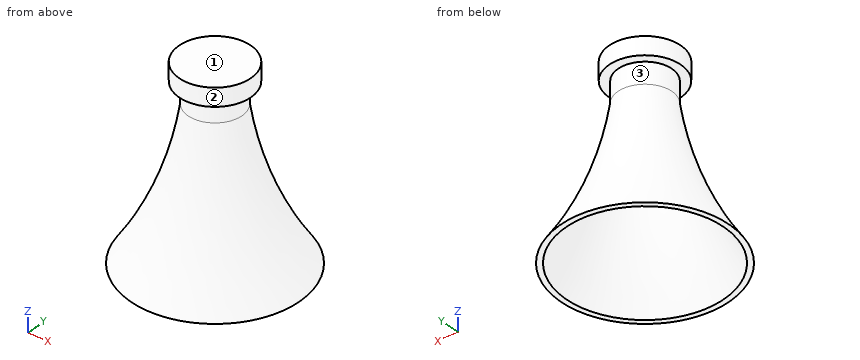
```python
from build123d import *


with BuildPart() as part:
    # Sketch1 → Revolve2 (revolve)
    with BuildSketch(Plane(origin=(0, 0, 0), x_dir=(1, 0, 0), z_dir=(0, 1, 0))):
        with BuildLine():
            ThreePointArc((9.415562128, 18.954471585), (5.262334896, 11.015891219), (3.004951609, 2.345563927))
            Line((3.004951609, 2.345563927), (3.004951609, 0))
            Line((3.004951609, 0), (4, 0))
            Line((4, 0), (4, -2))
            Line((4, -2), (0, -2))
            Line((0, -2), (0, 0))
            Line((0, 0), (0, 10))
            Line((0, 10), (0.75, 10))
            ThreePointArc((0.75, 10), (1.788096318, 6.210069956), (2.5, 2.345563927))
            ThreePointArc((2.5, 2.345563927), (4.722740089, 11.005000833), (8.813257881, 18.954471585))
            Line((8.813257881, 18.954471585), (9.415562128, 18.954471585))
        make_face()
    revolve(axis=Axis((0, 0, 2), (0, 0, -1)))


solid = part.part
```
The model under review builds one solid part; all positions refer to its coordinate system, in mm. Face numbers are marked on the shaded views. Round coordinates to 2 decimals unless told otherwise and drop trailing zeros. Loops run counter-clockwise (first coordinate to the right, second up) from the corner with the lowest first, then second, coordinate; pieces in that order, holes last.
1) Consider section A-A on z = -1.5. State the section outline as (x, y) points.
Values follow:
outline: circle Ø6.01 at (0, 0)
2) Consider section C-C on z = -8.5. Give the number of separate pieces and of enclosed holes in the cut face, then the cut area to 3 significant figures.
Values follow:
separate pieces: 2
enclosed holes: 1
area: 18.1 mm2
3) Wall thickness on line 1 along Y through (x, z) = (-1.5, -3.5); line 2 along X through (y, z) = (1.25, -6.5); line 3 along Y through (x, z) = (0, -8.75): over which ranges is each line inside the solid? List them lowest first.
Values follow:
line 1: y = -2.81 to -2.22, -1.77 to 1.77, 2.22 to 2.81
line 2: x = -3.61 to -3.06, -1.18 to 1.18, 3.06 to 3.61
line 3: y = -4.47 to -3.94, -1.13 to 1.13, 3.94 to 4.47
4) Consider section B-B on z = -15. State the section outline as (x, y) points.
Values follow:
outline: circle Ø14.12 at (0, 0); hole circle Ø12.99 at (0, 0)
5) Clearance check with flat-ended pins moving along their axes: P1, Ø2, axis at x = 6.5, z = -14, coming from the -Y side; P2, Ø1, axis at x = 7.5, y = 3.5, coming from the +Z side; P3, Ø1.6, axis at x = 0, y = 0.5, coming from the -Z side; P4, Ø1.5, axis at x = 6, z = -1, coming from the +Y side. State where each tip first meets the part, or that it passes through.
Values follow:
P1: stops at y = -3.82
P2: stops at z = -16.32
P3: stops at z = -10
P4: passes through
6) The part is to be moulded in two halves that separate along Z. For the marked faces 1, 2 and 3, say which applies: pulls with the +Z half, pulls with the -Z half, needs draft (parallel to the pull), parting line crosses it, or undercut.
Values follow:
face 1: pulls with the +Z half
face 2: needs draft
face 3: undercut
